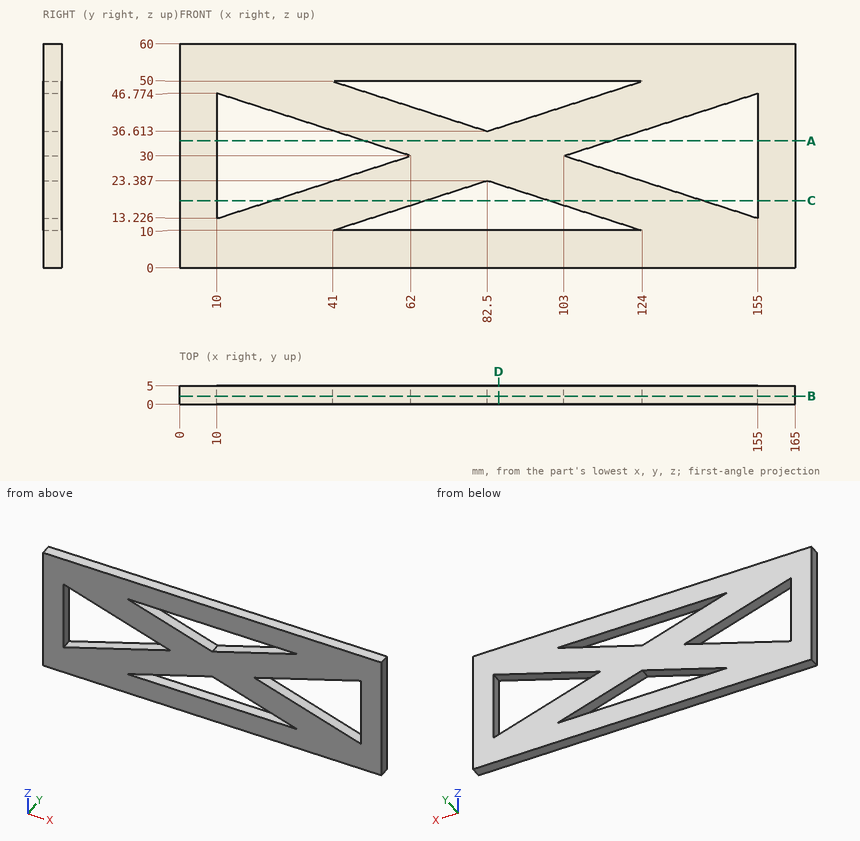
Check sheet for the drawn part. Datum: minimum x, y, z corner. Units: mm. Coordinates: 2 decimals unless noted, no trailing zeros. Loops run counter-clockwise (first coordinate to the right, second up) from the corner with the lowest first, then second, coordinate; pieces in that order, holes last. Notation, with made-up numbers: (27, 1) -> (41, 1) arc R29 cw to (41, 25) -> close; hole circle Ø8 at (18, -7.75). An arc over 180 degrees is marked (long way). Answer as CSV lines item,"result".
1) Cross-section at A-A, the plane z = 34. Record the cut outline in (x, y).
Found:
outline,"(0, 0) -> (10, 0) -> (10, 5) -> (0, 5) -> close; (49.6, 0) -> (115.4, 0) -> (115.4, 5) -> (49.6, 5) -> close; (155, 0) -> (165, 0) -> (165, 5) -> (155, 5) -> close"
2) Cross-section at D-D, the plane x = 85.5. Record the cut outline in (y, z), then the cut area to 3 significant figures.
Found:
outline,"(0, 0) -> (5, 0) -> (5, 10) -> (0, 10) -> close; (0, 22.42) -> (5, 22.42) -> (5, 37.58) -> (0, 37.58) -> close; (0, 50) -> (5, 50) -> (5, 60) -> (0, 60) -> close"
area,"176 mm2"
3) Thickness scan on L1, parallel to Z at x = 112, y = 4.35; L2, parallel to Z at x = 114, y = 3.2; L3, parallel to Z at x = 63, y = 0.2. Record the ranges inside material, lowest first. Write a range as from..to.
Found:
L1,"z = 0..10, 13.87..27.1, 32.9..46.13, 50..60"
L2,"z = 0..10, 13.23..26.45, 33.55..46.77, 50..60"
L3,"z = 0..10, 17.1..42.9, 50..60"
4) Cross-section at C-C, the plane z = 18. Record the cut outline in (x, y).
Found:
outline,"(0, 0) -> (10, 0) -> (10, 5) -> (0, 5) -> close; (24.8, 0) -> (65.8, 0) -> (65.8, 5) -> (24.8, 5) -> close; (99.2, 0) -> (140.2, 0) -> (140.2, 5) -> (99.2, 5) -> close; (155, 0) -> (165, 0) -> (165, 5) -> (155, 5) -> close"
5) Cross-section at B-B, the plane y = 2.25. Record the cut outline in (x, z).
Found:
outline,"(0, 0) -> (165, 0) -> (165, 60) -> (0, 60) -> close; hole (10, 13.23) -> (62, 30) -> (10, 46.77) -> close; hole (41, 10) -> (124, 10) -> (82.5, 23.39) -> close; hole (41, 50) -> (82.5, 36.61) -> (124, 50) -> close; hole (103, 30) -> (155, 13.23) -> (155, 46.77) -> close"
